Check sheet for the drawn part. Datum: minimum x, y, z corner. Units: mm. A direction names the side the tool comes from. Round coordinates to 2 decimals unless told otherwise and drop trailing zeros. Order: outer loops, then holes, each group sorted by start corner. A loop starts at its lowest first (then second) coordinate and runs counter-clockwise, first axis right, second up.
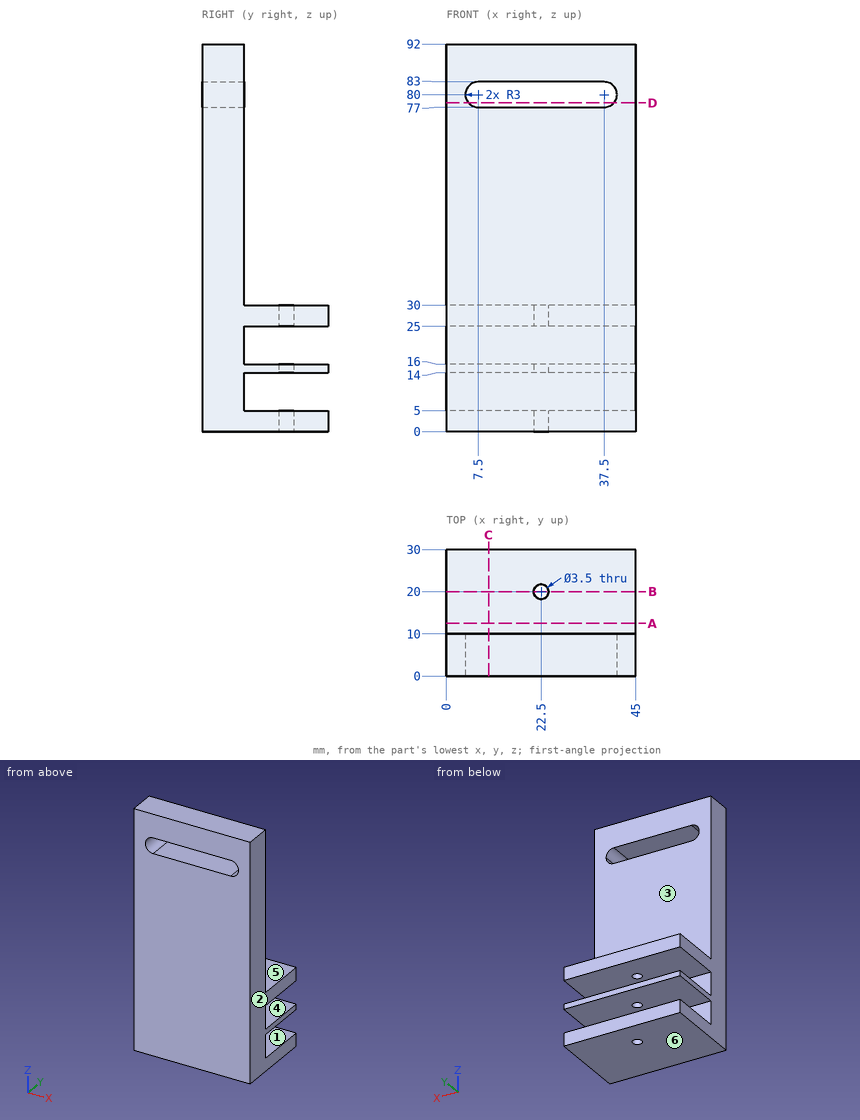
(1) Depth check by flat-ended pin: P1, Ø3, axis at x = 37, z = 72.5, coming from the +Y side; P2, Ø2, axis at x = 22.5, y = 20, coming from the +Z side; P3, Ø16, axis at x = 28, y = 25, coming from the +Z side. Enter the tip coordinate at first touch or a pass-through.
Returned:
P1: stops at y = 10
P2: passes through
P3: stops at z = 30
(2) Sectioned sample at B-B, the plane y = 20. Record the cut outline in (x, z), and give its area (3 significant figures).
Returned:
outline: (0, 0) - (20.75, 0) - (20.75, 5) - (0, 5) - close; (0, 14) - (20.75, 14) - (20.75, 16) - (0, 16) - close; (0, 25) - (20.75, 25) - (20.75, 30) - (0, 30) - close; (24.25, 0) - (45, 0) - (45, 5) - (24.25, 5) - close; (24.25, 14) - (45, 14) - (45, 16) - (24.25, 16) - close; (24.25, 25) - (45, 25) - (45, 30) - (24.25, 30) - close
area: 498 mm2
(3) Sectioned sample at D-D, the plane z = 78. Record the cut outline in (x, y), and give its area (3 significant figures).
Returned:
outline: (0, 0) - (5.26, 0) - (5.26, 10) - (0, 10) - close; (39.74, 0) - (45, 0) - (45, 10) - (39.74, 10) - close
area: 105 mm2
(4) Draft check along Z on the marked faces 4, 5 and 6. Enter one of: released by +Z, released by -Z, zero draft, split by the parting line, or undercut.
Returned:
face 4: undercut
face 5: released by +Z
face 6: released by -Z
(5) Sectioned sample at A-A, the plane y = 12.5. Record the cut outline in (x, z), and give its area (3 significant figures).
Returned:
outline: (0, 0) - (45, 0) - (45, 5) - (0, 5) - close; (0, 14) - (45, 14) - (45, 16) - (0, 16) - close; (0, 25) - (45, 25) - (45, 30) - (0, 30) - close
area: 540 mm2
(6) Set-up check for the marked faces 1, 2 and 3: record each of +Z, -Z, +X, -X, +Y, -Y from which the full face is reachable in a straight line by a thin tool's end or side.
Returned:
face 1: +X, -X, +Y
face 2: +Z, -Z, +X, +Y, -Y
face 3: +Z, +X, -X, +Y
(7) Sectioned sample at C-C, the plane x = 10. Record the cut outline in (y, z).
Returned:
outline: (0, 0) - (30, 0) - (30, 5) - (10, 5) - (10, 14) - (30, 14) - (30, 16) - (10, 16) - (10, 25) - (30, 25) - (30, 30) - (10, 30) - (10, 77) - (0, 77) - close; (0, 83) - (10, 83) - (10, 92) - (0, 92) - close
(8) Material ranges on line 1 (Z direction, x = 16, y = 13); line 2 (X direction, y = 20, z = 27.45); line 3 (Z direction, x = 36.5, y = 2.75), recorded low to high.
Returned:
line 1: z = 0 to 5, 14 to 16, 25 to 30
line 2: x = 0 to 20.75, 24.25 to 45
line 3: z = 0 to 77, 83 to 92
